from build123d import *

# Parameters (mm, degrees)
F0_W     = 200
F0_H     = 750
F1_DEPTH = 20
F2_W     = 200
F2_H     = 10
F3_DEPTH = 50
F4_W     = 200
F4_H     = 10
F5_DEPTH = 50
F6_W     = 200
F6_H     = 10
F7_DEPTH = 50
F8_W     = 200
F8_H     = 10
F9_DEPTH = 50


with BuildPart() as f1:
    # F0 (on Front) → F1 (new body)
    with BuildSketch(Plane.XZ):
        with Locations((-217.498518, 59.845)):
            Rectangle(F0_W, F0_H)
    extrude(amount=F1_DEPTH)

    # F2 (on Front) → F3 (join)
    with BuildSketch(Plane.XZ):
        with Locations((-218.074274, -100.155)):
            Rectangle(F2_W, F2_H)
    extrude(amount=-F3_DEPTH)

    # F4 (on Front) → F5 (join)
    with BuildSketch(Plane.XZ):
        with Locations((-217.498518, 79.845)):
            Rectangle(F4_W, F4_H)
    extrude(amount=-F5_DEPTH)

    # F6 (on Front) → F7 (join)
    with BuildSketch(Plane.XZ):
        with Locations((-217.498518, 259.845)):
            Rectangle(F6_W, F6_H)
    extrude(amount=-F7_DEPTH)

    # F8 (on Front) → F9 (join)
    with BuildSketch(Plane.XZ):
        with Locations((-217.498518, -280.155)):
            Rectangle(F8_W, F8_H)
    extrude(amount=-F9_DEPTH)


solid = f1.part
Read the model definition and answer for the solid it produces. Units are mm, in the model's axes. A direction names the side the tool comes from. Coordinates: 2 decimals unless noted, no trailing zeros. Loops run counter-clockwise (first coordinate to the right, second up) from the corner with the lowest first, then second, coordinate; pieces in that order, holes last.
Q1. The part is cut by section C-C on z = 233. Write down the section's boundary in (x, y), and give its area (3 significant figures).
Q2. Which of the six approach directions +Z, -Z, +X, -X, +Y, -Y give full straight-line access (tool end or side, diameter ignored) to faces 1 (the face through (-219, 0, 351)), 2 (the face through (-219, 0, 171)), 3 (the face through (-219, 25, -285.155))?
Q3. The part is cut by section B-B on x = -300.5. Write down the section's boundary in (y, z) (3 decimals), and give its area (3 significant figures).
Q4. The mould has two halves that part along Z. Classify faces 4 (the face through (-219, 25, 84.845)), 5 (the face through (-219, -20, 65)), 6 (the face through (-219, 25, 264.845)): +Z half, -Z half, draft (parallel to the pull), parting line (faces both ways), or undercut.
Q5. Each of these flat-tipped pins is pushed along its axis until it touches: pin 1 Ø25 at (x, y) = (-167.5, 23) entering from -Z (3 decimals); pin 2 Ø15 at (x, y) = (-192, 31) entering from +Z (3 decimals); pin 3 Ø5 at (y, z) = (36, -100) entering from +X. Where does it stop, or does it pass through?
Q6. Consider probe 1 along Z at (x, y) = (-196.5, 27.5) (3 decimals); probe 2 along Y at (x, z) = (-217.5, 295); probe 3 along X at (y, z) = (-0.5, 160). Determine where each line is inside the solid, lowest interval first.
Q7. The part is cut by section A-A on y = 27. Write down the section's boundary in (x, z) (3 decimals), and give its area (3 significant figures).
Results below:
1. outline: (-317.5, -20) - (-117.5, -20) - (-117.5, 0) - (-317.5, 0) - close
1. area: 4,000 mm2
2. face 1: +Z, +X, -X, +Y
2. face 2: +X, -X, +Y
2. face 3: -Z, +X, -X, +Y
3. outline: (-20, -315.155) - (0, -315.155) - (0, -285.155) - (50, -285.155) - (50, -275.155) - (0, -275.155) - (0, -105.155) - (50, -105.155) - (50, -95.155) - (0, -95.155) - (0, 74.845) - (50, 74.845) - (50, 84.845) - (0, 84.845) - (0, 254.845) - (50, 254.845) - (50, 264.845) - (0, 264.845) - (0, 434.845) - (-20, 434.845) - close
3. area: 17,000 mm2
4. face 4: undercut
4. face 5: draft
4. face 6: +Z half
5. pin 1: stops at z = -285.155
5. pin 2: stops at z = 264.845
5. pin 3: stops at x = -118.07
6. probe 1: z = -285.155 to -275.155, -105.155 to -95.155, 74.845 to 84.845, 254.845 to 264.845
6. probe 2: y = -20 to 0
6. probe 3: x = -317.5 to -117.5
7. outline: (-318.074, -105.155) - (-118.074, -105.155) - (-118.074, -95.155) - (-318.074, -95.155) - close; (-317.499, -285.155) - (-117.499, -285.155) - (-117.499, -275.155) - (-317.499, -275.155) - close; (-317.499, 74.845) - (-117.499, 74.845) - (-117.499, 84.845) - (-317.499, 84.845) - close; (-317.499, 254.845) - (-117.499, 254.845) - (-117.499, 264.845) - (-317.499, 264.845) - close
7. area: 8,000 mm2
